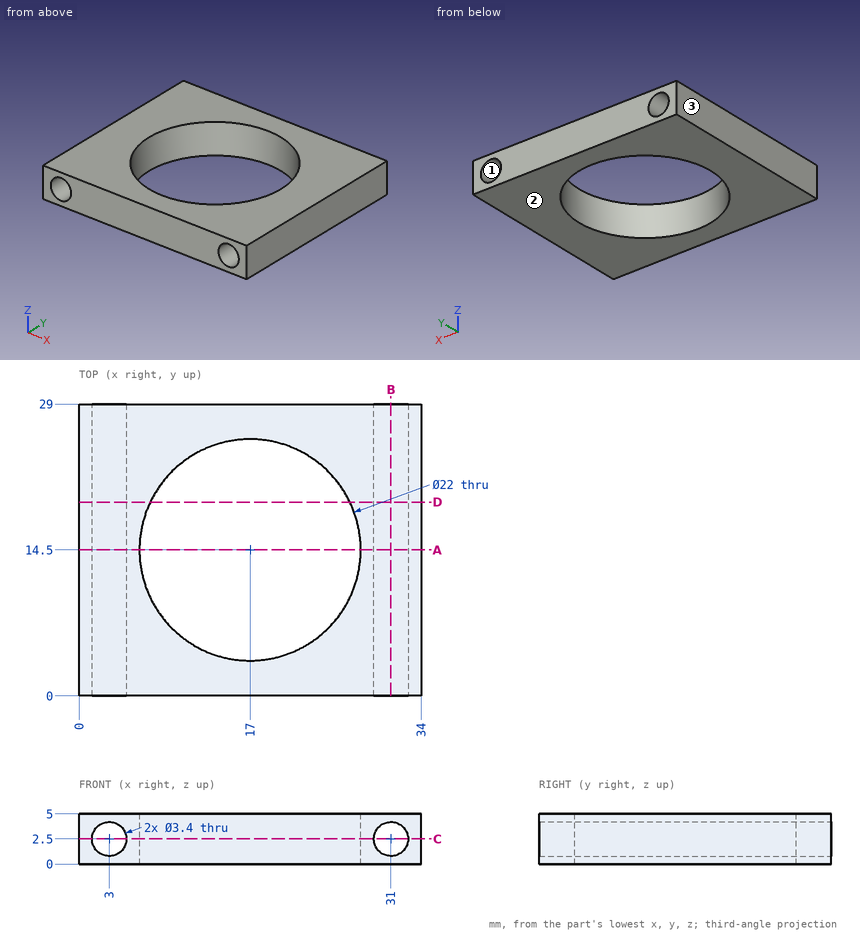
Study the drawing (mm; zero at the part's minimum x, y, z) and answer. Give positions to 0.01 mm unless a question says otherwise; leave off trailing zeros. Write each loop counter-clockwise with the first axis right and the second up, starting at its lowest first coordinate (ties: lowest second). Pieces come first, ordered by that corner, then holes. Notation, with made-up numbers: (27, 81.25) - (40, 81.25) arc R17 cw to (40, 106.25) - close; hole circle Ø1 at (49, 17). An arc over 180 degrees is marked (long way). Use a Markdown table: item, result.
1. Section A-A on y = 14.5 is taken. Write down the section's boundary in (x, z), plus the area to 3 significant figures.
Values follow:
| item | result |
|---|---|
| outline | (0, 0) - (6, 0) - (6, 5) - (0, 5) - close; (28, 0) - (34, 0) - (34, 5) - (28, 5) - close; hole circle Ø3.4 at (3, 2.5); hole circle Ø3.4 at (31, 2.5) |
| area | 41.8 mm² |
2. This flat-tipped pin is pushed along its axis until it touches: P1, Ø2, axis at x = 31, z = 2.5, coming from the +Y side. Where does it stop, or does it pass through?
Values follow:
| item | result |
|---|---|
| P1 | passes through |
3. For a pull along Z with two mould halves and no side action, classify the marked faces 1, 2 and 3 as released by +Z, released by -Z, zero draft, split by the parting line, or undercut.
Values follow:
| item | result |
|---|---|
| face 1 | undercut |
| face 2 | released by -Z |
| face 3 | zero draft |
4. Section D-D on y = 19.25 is taken. Write down the section's boundary in (x, z).
Values follow:
| item | result |
|---|---|
| outline | (0, 0) - (7.08, 0) - (7.08, 5) - (0, 5) - close; (26.92, 0) - (34, 0) - (34, 5) - (26.92, 5) - close; hole circle Ø3.4 at (3, 2.5); hole circle Ø3.4 at (31, 2.5) |
5. Section B-B on x = 31 is taken. Write down the section's boundary in (y, z), plus the area to 3 significant figures.
Values follow:
| item | result |
|---|---|
| outline | (0, 0) - (29, 0) - (29, 0.8) - (0, 0.8) - close; (0, 4.2) - (29, 4.2) - (29, 5) - (0, 5) - close |
| area | 46.4 mm² |
6. Find the intervals of material crossed by probe 1 along X at (y, z) = (12.5, 2.5); probe 2 along X at (y, z) = (7, 2.5); probe 3 along X at (y, z) = (2, 0.95), in increasing order. Write a range as from..to.
Values follow:
| item | result |
|---|---|
| probe 1 | x = 0..1.3, 4.7..6.18, 27.82..29.3, 32.7..34 |
| probe 2 | x = 0..1.3, 4.7..8.95, 25.05..29.3, 32.7..34 |
| probe 3 | x = 0..2.3, 3.7..30.3, 31.7..34 |
7. Section C-C on z = 2.5 is taken. Write down the section's boundary in (x, y).
Values follow:
| item | result |
|---|---|
| outline | (0, 0) - (1.3, 0) - (1.3, 29) - (0, 29) - close; (4.7, 0) - (29.3, 0) - (29.3, 29) - (4.7, 29) - close; (32.7, 0) - (34, 0) - (34, 29) - (32.7, 29) - close; hole circle Ø22 at (17, 14.5) |
